The drawing under review shows one solid part. Ordinate dimensions are in mm from its lowest x, y, z. A direction names the side the tool comes from. Coordinates: 2 decimals unless noted, no trailing zeros. Loops run counter-clockwise (first coordinate to the right, second up) from the corner with the lowest first, then second, coordinate; pieces in that order, holes last. Notation, with made-up numbers: M -0.5,-14 L 37.5,-14 A15 cw 37.5,8 Z; hole C 50.5,29 d5. An arc over 180 degrees is marked long. Return JSON: item names as keys, results as strings.
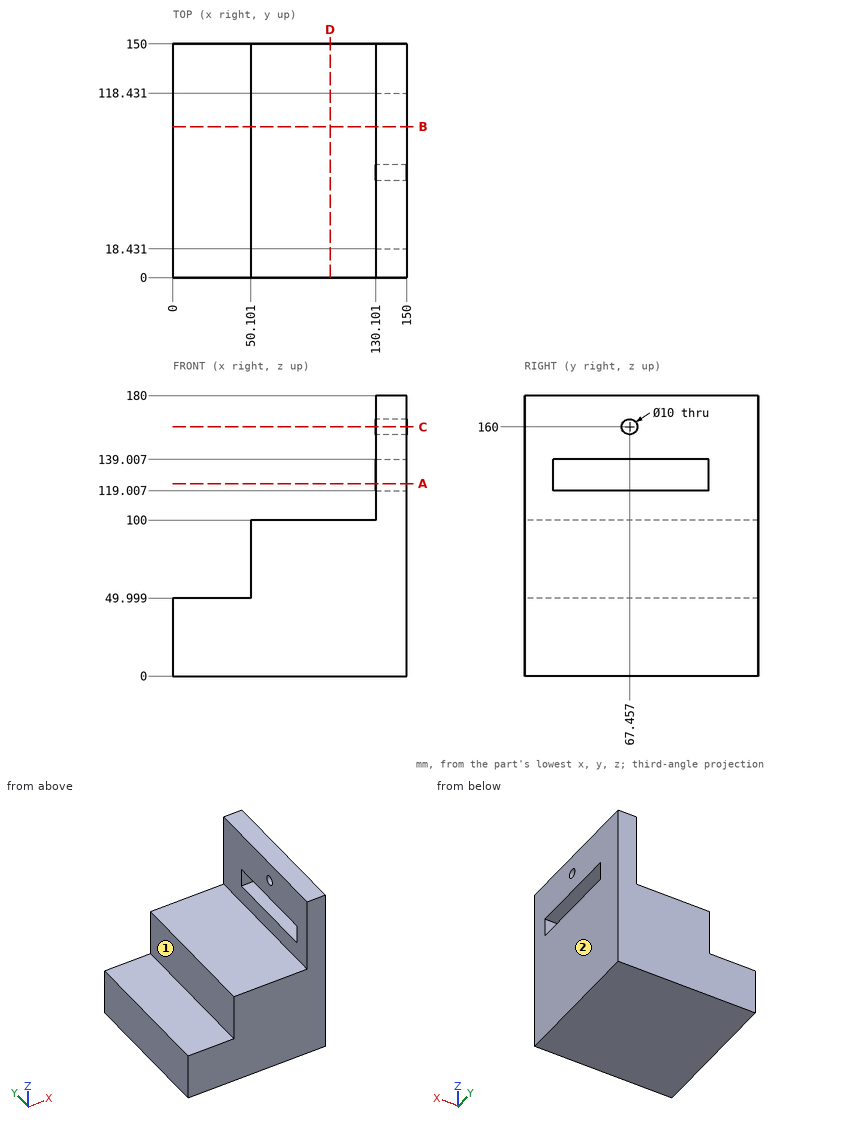
1. Add section A-A on z = 123.5. Give the boundary of the cut face in (x, y), plus the area to 3 significant figures.
Check values:
{"outline": "M 130.1,0 L 150,0 L 150,18.43 L 130.1,18.43 Z; M 130.1,118.43 L 150,118.43 L 150,150 L 130.1,150 Z", "area": "995 mm²"}
2. Machinability: for the marked faces 1 and 2, which of the approach directions +Z, -Z, +X, -X, +Y, -Y give a long, thin tool a straight path to every point of the face, cutting with its end or side? Answer none if there is none.
Check values:
{"face 1": "+Z, -X, +Y, -Y", "face 2": "+Z, -Z, +X, +Y, -Y"}
3. Insertion check: pin 1 Ø15 at (x, y) = (26.5, 82) entering from +Z; pin 2 Ø5 at (y, z) = (59, 155.5) entering from -X; pin 3 Ø10 at (x, y) = (59, 45.5) entering from +Z. Each pin has a flat end and moves straight along its axis. Give the tip position at first contact, or say it passes through.
Check values:
{"pin 1": "z = 50", "pin 2": "x = 130.1", "pin 3": "z = 100"}
4. Add section B-B on y = 97. Give the boundary of the cut face in (x, z).
Check values:
{"outline": "M 0,0 L 150,0 L 150,119.01 L 130.1,119.01 L 130.1,100 L 50.1,100 L 50.1,50 L 0,50 Z; M 130.1,139.01 L 150,139.01 L 150,180 L 130.1,180 Z"}
5. Add section D-D on x = 101. Give the boundary of the cut face in (y, z).
Check values:
{"outline": "M 0,0 L 150,0 L 150,100 L 0,100 Z"}
6. To check wall thickness, follow line 1 (Y direction, x = 141, z = 160); line 2 (X direction, y = 92, z = 169); line 3 (X direction, y = 53.5, z = 98). State the ranges of each line that lie inside material, in increasing order.
Check values:
{"line 1": "0 to 62.46, 72.46 to 150", "line 2": "130.1 to 150", "line 3": "50.1 to 150"}
7. Add section C-C on z = 160. Give the boundary of the cut face in (x, y), plus the area to 3 significant figures.
Check values:
{"outline": "M 130.1,0 L 150,0 L 150,62.46 L 130.1,62.46 Z; M 130.1,72.46 L 150,72.46 L 150,150 L 130.1,150 Z", "area": "2,790 mm²"}
